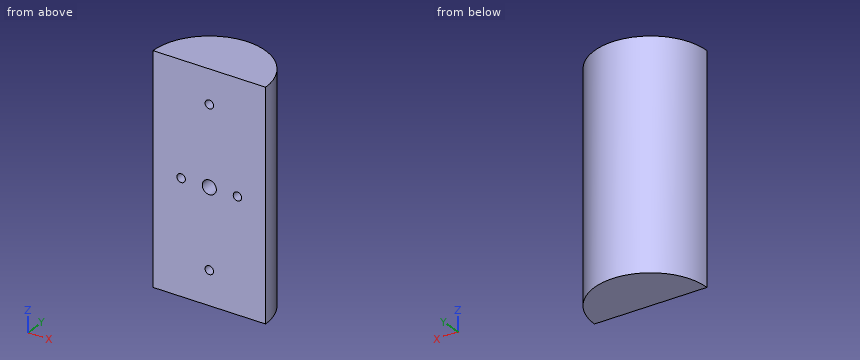
Autodesk Inventor part; units mm, degrees
ref_plane "YZ Plane" through (0, 0, 0) normal (1, 0, 0) x (0, 1, 0)
ref_plane "XZ Plane" through (0, 0, 0) normal (0, 1, 0) x (-1, 0, 0)
ref_plane "XY Plane" through (0, 0, 0) normal (0, 0, 1) x (1, 0, 0)
sketch "Sketch1" plane through (0, 0, 0) normal (0, 0, 1) x (1, 0, 0)
  arc A0 (31.75, 0) -> (-31.75, 0) centre (0, 0) ccw
  line L0 (-31.75, 0) -> (31.75, 0)
  dimension "diameter" = 63.5
extrude "Extrusion1" add sketch "Sketch1" along normal blind 127
sketch "Sketch2" plane through (-31.75, 0, 0) normal (0, -1, 0) x (1, 0, 0)
  line L0 (31.75, 0) -> (31.75, 127) construction
  line L1 (0, 127) -> (63.5, 127) construction
  line L2 (0, 0) -> (0, 127) construction
  line L3 (0, 63.5) -> (63.5, 63.5) construction
  line L4 (63.5, 0) -> (63.5, 127) construction
  point P0 (31.75, 63.5)
  point P1 (31.75, 107.95)
  point P2 (31.75, 19.05)
  point P3 (47.625, 63.5)
  point P4 (15.875, 63.5)
  dimension "d3" = 44.45
  dimension "d4" = 44.45
  dimension "d12" = 15.875
hole "Hole1" at (0, 0, 107.95) at (0, 0, 19.05) at (15.875, 0, 63.5) at (-15.875, 0, 63.5) direction (0, 1, 0) diameter 4.7625 depth 6.35
hole "Hole2" at (0, 0, 63.5) direction (0, 1, 0) diameter 7.9375 depth 12.7
equation "\"width\" = 2 * diameter"
properties part number "Greenhouse_3DPrint"
Check sheet for the modelled part. Datum: model origin and axes. Units: mm. Round coordinates to 2 decimals unless told otherwise and drop trailing zeros. Order: outer loops, then holes, each group sorted by start corner. A loop starts at its lowest first (then second) coordinate and runs counter-clockwise, first axis right, second up. Notation, with made-up numbers: (86, 37.25) -> (145, 37.25) arc R14 ccw to (145, 62.25) -> close; hole circle Ø5 at (6.5, -24). An arc over 180 degrees is marked (long way). One line per item, written item: value. Start each with the question number.
Q1. Cross-section at C-C (y = 10.5). Record the boundary of the cut face in (x, z).
Q2. Cross-section at D-D (z = 107.95). Record the boundary of the cut face in (x, y), and give its area (3 significant figures).
Q3. Gauge pin test, flat ends, axial feed: pin 1 Ø6.5 at (x, z) = (0, 63.5) entering from +Y; pin 2 Ø4 at (x, z) = (0, 19) entering from -Y; pin 3 Ø5 at (y, z) = (21, 81.5) entering from +X. Record the tip position at first contact, or that the pin passes through.
Q4. Cross-section at A-A (z = 63.5). Record the boundary of the cut face in (x, y).
Q5. Cross-section at B-B (x = 0). Record the boundary of the cut face in (y, z).
Q6. Thickness scan on line 1 (Z direction, x = 0, y = 4.25); line 2 (X direction, y = 2, z = 63); line 3 (X direction, y = 3, z = 63). Record the ranges inside material, lowest first.
Completed:
1. outline: (-29.96, 0) -> (29.96, 0) -> (29.96, 127) -> (-29.96, 127) -> close; hole circle Ø7.94 at (0, 63.5)
2. outline: (-31.75, 0) -> (-2.38, 0) -> (-2.38, 6.35) -> (2.38, 6.35) -> (2.38, 0) -> (31.75, 0) arc R31.75 ccw to start
2. area: 1,550 mm²
3. pin 1: stops at y = 31.75
3. pin 2: stops at y = 6.35
3. pin 3: stops at x = 25.8
4. outline: (-31.75, 0) -> (-18.26, 0) -> (-18.26, 6.35) -> (-13.49, 6.35) -> (-13.49, 0) -> (-3.97, 0) -> (-3.97, 12.7) -> (3.97, 12.7) -> (3.97, 0) -> (13.49, 0) -> (13.49, 6.35) -> (18.26, 6.35) -> (18.26, 0) -> (31.75, 0) arc R31.75 ccw to start
5. outline: (0, 0) -> (31.75, 0) -> (31.75, 127) -> (0, 127) -> (0, 110.33) -> (6.35, 110.33) -> (6.35, 105.57) -> (0, 105.57) -> (0, 67.47) -> (12.7, 67.47) -> (12.7, 59.53) -> (0, 59.53) -> (0, 21.43) -> (6.35, 21.43) -> (6.35, 16.67) -> (0, 16.67) -> close
6. line 1: z = 0 to 16.67, 21.43 to 59.53, 67.47 to 105.57, 110.33 to 127
6. line 2: x = -31.69 to -18.2, -13.55 to -3.94, 3.94 to 13.55, 18.2 to 31.69
6. line 3: x = -31.61 to -18.2, -13.55 to -3.94, 3.94 to 13.55, 18.2 to 31.61
